Design review of the part built by this model. Coordinates are the model's own, in mm. Face numbers are marked on the shaded views. A direction names the side the tool comes from. Coordinates: 2 decimals unless noted, no trailing zeros. Loops run counter-clockwise (first coordinate to the right, second up) from the corner with the lowest first, then second, coordinate; pieces in that order, holes last.
from build123d import *

# Parameters (mm, degrees)
BOSS_EXTRUDE1_DEPTH   = 20
BOSS_EXTRUDE1_2_DEPTH = 20
BOSS_EXTRUDE2_DEPTH   = 20
CUT_EXTRUDE1_DEPTH    = 7.5
SKETCH3_R             = 1.75
CUT_EXTRUDE2_DEPTH    = 27.369487129


with BuildPart() as part:
    # Sketch2 → Boss-Extrude1 (new, symmetric)
    with BuildSketch(Plane.XY):
        with BuildLine():
            ThreePointArc((8.364209467, 2), (8.540848945, 1.006925665), (8.6, 0))
            Line((8.6, 0), (16.364209467, 0))
            Line((16.364209467, 0), (16.364209467, 2))
            Line((16.364209467, 2), (8.364209467, 2))
        make_face()
    extrude(amount=BOSS_EXTRUDE1_DEPTH, both=True)



with BuildPart() as body_2:
    # Sketch2 → Boss-Extrude1 2 (new, symmetric)
    with BuildSketch(Plane.XY):
        with BuildLine():
            Line((-16.364209467, 0), (-8.6, 0))
            ThreePointArc((-8.6, 0), (-8.540848945, 1.006925665), (-8.364209467, 2))
            Line((-8.364209467, 2), (-16.364209467, 2))
            Line((-16.364209467, 2), (-16.364209467, 0))
        make_face()
    extrude(amount=BOSS_EXTRUDE1_2_DEPTH, both=True)


with BuildPart() as part_1:
    add(part.part)

    add(body_2.part)  # Boss-Extrude2 merges body 2
    # Sketch2_4 → Boss-Extrude2 (add, symmetric)
    with BuildSketch(Plane.XY):
        with BuildLine():
            Line((8.6, 0), (6.6, 0))
            ThreePointArc((6.6, 0), (5.914302048, 2.929339736), (3.999687488, 5.25))
            Line((3.999687488, 5.25), (-3.999687488, 5.25))
            ThreePointArc((-3.999687488, 5.25), (-5.914302048, 2.929339736), (-6.6, 0))
            Line((-6.6, 0), (-8.6, 0))
            ThreePointArc((-8.6, 0), (-7.541266186, 4.133921179), (-4.625743184, 7.25))
            Line((-4.625743184, 7.25), (4.625743184, 7.25))
            ThreePointArc((4.625743184, 7.25), (7.541266186, 4.133921179), (8.6, 0))
        make_face()
    extrude(amount=BOSS_EXTRUDE2_DEPTH, both=True)

    # Sketch2_5 → Cut-Extrude1 (cut, symmetric)
    with BuildSketch(Plane.XY):
        with BuildLine():
            Line((8.6, 0), (6.6, 0))
            ThreePointArc((6.6, 0), (5.914302048, 2.929339736), (3.999687488, 5.25))
            Line((3.999687488, 5.25), (-3.999687488, 5.25))
            ThreePointArc((-3.999687488, 5.25), (-5.914302048, 2.929339736), (-6.6, 0))
            Line((-6.6, 0), (-8.6, 0))
            ThreePointArc((-8.6, 0), (-7.541266186, 4.133921179), (-4.625743184, 7.25))
            Line((-4.625743184, 7.25), (4.625743184, 7.25))
            ThreePointArc((4.625743184, 7.25), (7.541266186, 4.133921179), (8.6, 0))
        make_face()
    extrude(amount=CUT_EXTRUDE1_DEPTH, both=True, mode=Mode.SUBTRACT)

    # Sketch3 → Cut-Extrude2 (cut, through all)
    with BuildSketch(Plane(origin=(0, 2, 0), x_dir=(1, 0, 0), z_dir=(0, 1, 0))):
        with Locations(Location((-13.364209467, 15, 0), (0, 0, 270))):
            Circle(SKETCH3_R)
        with Locations(Location((-13.364209467, -15, 0), (0, 0, 270))):
            Circle(SKETCH3_R)
    cut_extrude2 = extrude(amount=-CUT_EXTRUDE2_DEPTH, mode=Mode.SUBTRACT)

    # Mirror1: Cut-Extrude2 across plane
    add(cut_extrude2.mirror(Plane(origin=(0, 0, 0), x_dir=(0, 0, 1), z_dir=(1, 0, 0))), mode=Mode.SUBTRACT)


solid = part_1.part
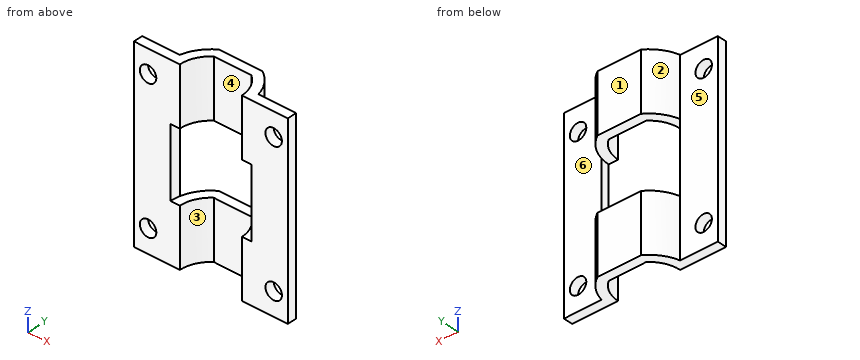
Q1. Take a section at C-C, the plane z = -15. Write out the cut boundary in (x, y), then the cut area to 3 significant figures.
Q2. Machinability: for the marked faces 4, 5 and 6, which of the approach directions +Z, -Z, +X, -X, +Y, -Y give a long, thin tool a straight path to every point of the face, cutting with its end or side? Answer none if there is none.
Q3. Take a section at D-D, the plane y = 0.5. Write out the cut boundary in (x, z), then the cut area to 3 significant figures.
Q4. Take a section at A-A, the plane x = -3. Write out the cut boundary in (y, z), then the cut area to 3 significant figures.
Q5. The part is to be moulded in two halves that separate along X. For the marked faces 1, 2 and 3, say which applies: pulls with the +X half, pulls with the -X half, needs draft (parallel to the pull), parting line crosses it, or undercut.
Q6. Clearance check with flat-ended pins moving along their axes: pin 1 Ø6.5 at (x, z) = (1, -14.5) entering from -Y; pin 2 Ø2.5 at (x, z) = (-11.5, -7.5) entering from +Y; pin 3 Ø4 at (x, z) = (1.5, 14.5) entering from -Y. State where each tip first meets the part, or that it passes through.
Q7. Take a section at B-B, the plane z = 7. Write out the cut boundary in (x, y), then the cut area to 3 significant figures.
Q8. For line 1 (Z direction, x = -3, y = 6); line 2 (X direction, y = 0.75, z = 14); line 3 (X direction, y = 0.6, z = -15), list the stretches that pass through material, from the lowest coordinate up.
Entries:
1. outline: (-16.36, 0) - (-15.11, 0) - (-15.11, 2) - (-16.36, 2) - close; (-11.61, 0) - (-6.6, 0) arc R6.6 cw to (-4, 5.25) - (4, 5.25) arc R6.6 cw to (6.6, 0) - (11.61, 0) - (11.61, 2) - (8.36, 2) arc R8.6 ccw to (4.63, 7.25) - (-4.63, 7.25) arc R8.6 ccw to (-8.36, 2) - (-11.61, 2) - close; (15.11, 0) - (16.36, 0) - (16.36, 2) - (15.11, 2) - close
1. area: 64.0 mm2
2. face 4: +Z, -Z, -Y
2. face 5: +Z, -Z, -X, +Y
2. face 6: +Z, -Z, +X, +Y
3. outline: (-16.36, -20) - (-6.58, -20) - (-6.58, -7.5) - (-8.59, -7.5) - (-8.59, 7.5) - (-6.58, 7.5) - (-6.58, 20) - (-16.36, 20) - close; (6.58, -20) - (16.36, -20) - (16.36, 20) - (6.58, 20) - (6.58, 7.5) - (8.59, 7.5) - (8.59, -7.5) - (6.58, -7.5) - close; hole circle Ø3.5 at (-13.36, -15); hole circle Ø3.5 at (-13.36, 15); hole circle Ø3.5 at (13.36, -15); hole circle Ø3.5 at (13.36, 15)
3. area: 684 mm2
4. outline: (5.25, -20) - (7.25, -20) - (7.25, -7.5) - (5.25, -7.5) - close; (5.25, 7.5) - (7.25, 7.5) - (7.25, 20) - (5.25, 20) - close
4. area: 50.0 mm2
5. face 1: needs draft
5. face 2: pulls with the -X half
5. face 3: undercut
6. pin 1: stops at y = 5.05
6. pin 2: stops at y = 2
6. pin 3: stops at y = 5.25
7. outline: (-16.36, 0) - (-8.6, 0) arc R8.6 cw to (-8.36, 2) - (-16.36, 2) - close; (8.36, 2) arc R8.6 cw to (8.6, 0) - (16.36, 0) - (16.36, 2) - close
7. area: 31.4 mm2
8. line 1: z = -20 to -7.5, 7.5 to 20
8. line 2: x = -16.36 to -14.8, -11.93 to -6.56, 6.56 to 11.93, 14.8 to 16.36
8. line 3: x = -16.36 to -15.11, -11.61 to -6.57, 6.57 to 11.61, 15.11 to 16.36
